```python
from build123d import *

# Parameters (mm, degrees)
F1_DEPTH  = 38.1
F3_DEPTH  = 3.175
F4_R      = 7.9375
F5_R      = 6.35
F9_R      = 12.7
F10_R     = 1.905
F11_DEPTH = 3.176


# Not quite as in the source:
# - a pattern or mirror of a feature is missing from the dataset's text; its kind, count and spacing are read off the source's solid


with BuildPart() as f1:
    # F0 (on Top) → F1 (new body)
    with BuildSketch(Plane.XY):
        Polygon((0, -34.925), (0, 0), (34.925, 0), (34.925, 3.175), (-3.175, 3.175), (-3.175, -34.925), align=None)
    extrude(amount=-F1_DEPTH)

    # F2 (on face) → F3 (join)
    with BuildSketch(Plane.XY):
        Polygon((6.35, -34.925), (6.35, -6.35), (34.925, -6.35), (34.925, 3.175), (-3.175, 3.175), (-3.175, -34.925), align=None)
    extrude(amount=F3_DEPTH)

    # F4
    f4_edges = [f1.edges().sort_by_distance(p)[0] for p in [
        (6.35, -6.35, 1.5875),
    ]]
    fillet(f4_edges, radius=F4_R)

    # F5
    f5_edges = [f1.edges().sort_by_distance(p)[0] for p in [
        (6.35, -34.925, 1.5875),
        (34.925, -6.35, 1.5875),
    ]]
    fillet(f5_edges, radius=F5_R)

    # F9
    f9_edges = [f1.edges().sort_by_distance(p)[0] for p in [
        (34.925, 1.5875, -38.1),
        (-1.5875, -34.925, -38.1),
    ]]
    fillet(f9_edges, radius=F9_R)

    # F10 (on face) → F11 (cut, through all)
    with BuildSketch(Plane.XZ):
        with Locations((17.4625, -19.05)):
            Circle(F10_R)
    f11 = extrude(amount=-F11_DEPTH, mode=Mode.SUBTRACT)

    # F11_copies: F11 across plane
    add(f11.mirror(Plane(origin=(0, 0, 0), x_dir=(0.7071067812, -0.7071067812, 0), z_dir=(-0.7071067812, -0.7071067812, 0))), mode=Mode.SUBTRACT)


solid = f1.part
```
Can you work these out from the model? Positions are in its coordinate system, mm. A direction names the side the tool comes from. Give positions to 0.01 mm unless a question says otherwise; leave off trailing zeros. Order: outer loops, then holes, each group sorted by start corner. A loop starts at its lowest first (then second) coordinate and runs counter-clockwise, first axis right, second up. Notation, with made-up numbers: M -7.75,-31 L 40.25,-31 A4 cw 40.25,-25 Z; hole C 23,-39.75 d1. An arc over 180 degrees is marked long. One line per item, written item: value.
1) I want a section at A-A, the plane z = -19.05. List the corners of the cut face in (x, y) for me (1 decimal).
Answer sheet:
outline: M -3.2,-34.9 L 0,-34.9 L 0,-19.4 L -3.2,-19.4 Z; M -3.2,-15.6 L 0,-15.6 L 0,0 L 15.6,0 L 15.6,3.2 L -3.2,3.2 Z; M 19.4,0 L 34.9,0 L 34.9,3.2 L 19.4,3.2 Z
2) Please list where these lines run through material, in increasing order: line 1 along Y through (x, z) = (-2, -19) (3 decimals); line 2 along Z through (x, y) = (1.5, -0.5) (3 decimals).
Answer sheet:
line 1: y = -34.925 to -19.367, -15.558 to 3.175
line 2: z = 0 to 3.175
3) On a 3-axis mill with a long thin cutter (end or side, diameter ignored), from which of +Z, -Z, +X, -X, +Y, -Y can I reach the whole of each face in a straight line? I mean faces 5 (the face through (-1.57, -19.28, -18.48)), 6 (the face through (6.35, -22, 2)), 7 (the face through (6, -9, 0)). Say none if no direction works.
Answer sheet:
face 5: +X, -X
face 6: +Z, -Z, +X, -Y
face 7: -Z, +X, -Y
4) I want a section at B-B, the plane y = -3.5. List the corners of the cut face in (x, z) for me (3 decimals).
Answer sheet:
outline: M -3.175,-38.1 L 0,-38.1 L 0,0 L 33.873,0 L 33.873,3.175 L -3.175,3.175 Z
5) We'd pull the mould along X, two halves only. Please class faces 1 (the face through (-3.175, -15.6, -17.8)), 2 (the face through (12, 3.175, -18)), 3 (the face through (18.487, 1.565, -17.444)), 4 (the face through (4.539, -33.015, 1.61)): released by +X, released by -X, zero draft, split by the parting line, or undercut.
Answer sheet:
face 1: released by -X
face 2: zero draft
face 3: undercut
face 4: released by +X
6) For P1, Ø8, axis at y = -23.5, z = -18.5, coming from the +X side; P2, Ø6, axis at x = 25.5, z = -20.5, coming from the -Y side; P3, Ø1, axis at x = 21.5, z = 2.5, coming from the -Y side; P4, Ø2.5, axis at y = -17.46, z = -19.05, coming from the +X side (1 decimal), each with a flat end and sliding along its axis, tell me the tip position at first contact or that it passes through.
Answer sheet:
P1: stops at x = 0
P2: stops at y = 0
P3: stops at y = -6.35
P4: passes through
7) I want a section at C-C, the plane x = 11.5. List the corners of the cut face in (y, z) for me (3 decimals).
Answer sheet:
outline: M -6.856,0 L 0,0 L 0,-38.1 L 3.175,-38.1 L 3.175,3.175 L -6.856,3.175 Z
